Can you work these out from the model? Positions are in its coordinate system, mm. A direction names the side the tool comes from. Give positions to 0.01 mm unless a question says otherwise; leave off trailing zeros. One line per question, with ' | ' between items.
from build123d import *

# Parameters (mm, degrees)
SKETCH1_W             = 25.4
SKETCH1_H             = 25.4
SKETCH1_W_2           = 23.4
SKETCH1_H_2           = 23.4
BOSS_EXTRUDE1_DEPTH   = 304.8
BOSS_EXTRUDE1_2_DEPTH = 304.8
BOSS_EXTRUDE1_3_DEPTH = 304.8
BOSS_EXTRUDE1_4_DEPTH = 304.8
SKETCH2_W             = 25.4
SKETCH2_H             = 25.4
SKETCH2_W_2           = 23.4
SKETCH2_H_2           = 23.4
BOSS_EXTRUDE2_DEPTH   = 508
SKETCH3_W             = 25.4
SKETCH3_H             = 25.4
SKETCH3_W_2           = 23.4
SKETCH3_H_2           = 23.4
BOSS_EXTRUDE4_DEPTH   = 254
LPATTERN2_COUNT       = 2
LPATTERN2_PITCH       = 279.4
SKETCH4_W             = 25.4
SKETCH4_H             = 50.8
SKETCH4_W_2           = 23.4
SKETCH4_H_2           = 48.8
BOSS_EXTRUDE5_DEPTH   = 101.6
SKETCH5_W             = 25.4
SKETCH5_H             = 25.4
SKETCH5_W_2           = 23.4
SKETCH5_H_2           = 23.4
BOSS_EXTRUDE6_DEPTH   = 635
LPATTERN3_COUNT       = 2
LPATTERN3_PITCH       = 660.4
LPATTERN4_COUNT       = 2
LPATTERN4_PITCH       = 736.6


with BuildPart() as part:
    # Sketch1 → Boss-Extrude1 (new body)
    with BuildSketch(Plane(origin=(0, 0, 0), x_dir=(1, 0, 0), z_dir=(0, 1, 0))):
        with Locations((139.7, 266.7)):
            Rectangle(SKETCH1_W, SKETCH1_H)
        with Locations((139.7, 266.7)):
            Rectangle(SKETCH1_W_2, SKETCH1_H_2, mode=Mode.SUBTRACT)
    extrude(amount=BOSS_EXTRUDE1_DEPTH)



with BuildPart() as body_2:
    # Sketch1 → Boss-Extrude1 2 (new body)
    with BuildSketch(Plane(origin=(0, 0, 0), x_dir=(1, 0, 0), z_dir=(0, 1, 0))):
        with Locations((139.7, -266.7)):
            Rectangle(SKETCH1_W, SKETCH1_H)
        with Locations((139.7, -266.7)):
            Rectangle(SKETCH1_W_2, SKETCH1_H_2, mode=Mode.SUBTRACT)
    extrude(amount=BOSS_EXTRUDE1_2_DEPTH)


with BuildPart() as body_3:
    # Sketch1 → Boss-Extrude1 3 (new body)
    with BuildSketch(Plane(origin=(0, 0, 0), x_dir=(1, 0, 0), z_dir=(0, 1, 0))):
        with Locations((-139.7, -266.7)):
            Rectangle(SKETCH1_W, SKETCH1_H)
        with Locations((-139.7, -266.7)):
            Rectangle(SKETCH1_W_2, SKETCH1_H_2, mode=Mode.SUBTRACT)
    extrude(amount=BOSS_EXTRUDE1_3_DEPTH)


with BuildPart() as body_4:
    # Sketch1 → Boss-Extrude1 4 (new body)
    with BuildSketch(Plane(origin=(0, 0, 0), x_dir=(1, 0, 0), z_dir=(0, 1, 0))):
        with Locations((-139.7, 266.7)):
            Rectangle(SKETCH1_W, SKETCH1_H)
        with Locations((-139.7, 266.7)):
            Rectangle(SKETCH1_W_2, SKETCH1_H_2, mode=Mode.SUBTRACT)
    extrude(amount=BOSS_EXTRUDE1_4_DEPTH)


with BuildPart() as part_1:
    add(part.part)

    add(body_2.part)  # Boss-Extrude2 merges body 2
    # Sketch2 → Boss-Extrude2 (add)
    # profile 1 of 2: a face of its own
    with BuildSketch(Plane.XY.offset(-254)):
        with Locations((139.7, 292.1)):
            Rectangle(SKETCH2_W, SKETCH2_H)
        with Locations((139.7, 292.1)):
            Rectangle(SKETCH2_W_2, SKETCH2_H_2, mode=Mode.SUBTRACT)
    # profile 2 of 2: a face of its own
    with BuildSketch(Plane.XY.offset(-254)):
        with Locations((139.7, 12.7)):
            Rectangle(SKETCH2_W, SKETCH2_H)
        with Locations((139.7, 12.7)):
            Rectangle(SKETCH2_W_2, SKETCH2_H_2, mode=Mode.SUBTRACT)
    boss_extrude2 = extrude(amount=BOSS_EXTRUDE2_DEPTH)


    add(body_3.part)  # Boss-Extrude4 merges body 3

    add(body_4.part)  # Boss-Extrude4 merges body 4
    # Sketch3 → Boss-Extrude4 (add)
    # profile 1 of 4: a face of its own
    with BuildSketch(Plane.ZY.offset(-127)):
        with Locations((266.7, 292.1)):
            Rectangle(SKETCH3_W, SKETCH3_H)
        with Locations((266.7, 292.1)):
            Rectangle(SKETCH3_W_2, SKETCH3_H_2, mode=Mode.SUBTRACT)
    # profile 2 of 4: a face of its own
    with BuildSketch(Plane.ZY.offset(-127)):
        with Locations((-266.7, 292.1)):
            Rectangle(SKETCH3_W, SKETCH3_H)
        with Locations((-266.7, 292.1)):
            Rectangle(SKETCH3_W_2, SKETCH3_H_2, mode=Mode.SUBTRACT)
    # profile 3 of 4: a face of its own
    with BuildSketch(Plane.ZY.offset(-127)):
        with Locations((266.7, 12.7)):
            Rectangle(SKETCH3_W, SKETCH3_H)
        with Locations((266.7, 12.7)):
            Rectangle(SKETCH3_W_2, SKETCH3_H_2, mode=Mode.SUBTRACT)
    # profile 4 of 4: a face of its own
    with BuildSketch(Plane.ZY.offset(-127)):
        with Locations((-266.7, 12.7)):
            Rectangle(SKETCH3_W, SKETCH3_H)
        with Locations((-266.7, 12.7)):
            Rectangle(SKETCH3_W_2, SKETCH3_H_2, mode=Mode.SUBTRACT)
    extrude(amount=BOSS_EXTRUDE4_DEPTH)

    # LPattern2: Boss-Extrude2 ×2
    with Locations(*[(-i * LPATTERN2_PITCH, 0, 0) for i in range(1, LPATTERN2_COUNT)]):
        add(boss_extrude2)

    # Sketch4 → Boss-Extrude5 (add)
    # profile 1 of 2: a face of its own
    with BuildSketch(Plane(origin=(0, 0, -279.4), x_dir=(-1, 0, 0), z_dir=(0, 0, -1))):
        with Locations((-139.7, 25.4)):
            Rectangle(SKETCH4_W, SKETCH4_H)
        with Locations((-139.7, 25.4)):
            Rectangle(SKETCH4_W_2, SKETCH4_H_2, mode=Mode.SUBTRACT)
    # profile 2 of 2: a face of its own
    with BuildSketch(Plane(origin=(0, 0, -279.4), x_dir=(-1, 0, 0), z_dir=(0, 0, -1))):
        with Locations((139.7, 25.4)):
            Rectangle(SKETCH4_W, SKETCH4_H)
        with Locations((139.7, 25.4)):
            Rectangle(SKETCH4_W_2, SKETCH4_H_2, mode=Mode.SUBTRACT)
    boss_extrude5 = extrude(amount=BOSS_EXTRUDE5_DEPTH)

    # Sketch5 → Boss-Extrude6 (add)
    # profile 1 of 2: a face of its own
    with BuildSketch(Plane.XZ):
        with Locations((-139.7, -368.3)):
            Rectangle(SKETCH5_W, SKETCH5_H)
        with Locations((-139.7, -368.3)):
            Rectangle(SKETCH5_W_2, SKETCH5_H_2, mode=Mode.SUBTRACT)
    # profile 2 of 2: a face of its own
    with BuildSketch(Plane.XZ):
        with Locations((139.7, -368.3)):
            Rectangle(SKETCH5_W, SKETCH5_H)
        with Locations((139.7, -368.3)):
            Rectangle(SKETCH5_W_2, SKETCH5_H_2, mode=Mode.SUBTRACT)
    boss_extrude6 = extrude(amount=BOSS_EXTRUDE6_DEPTH)

    # LPattern3: Boss-Extrude5 ×2
    with Locations(*[(0, 0, i * LPATTERN3_PITCH) for i in range(1, LPATTERN3_COUNT)]):
        add(boss_extrude5)

    # LPattern4: Boss-Extrude6 ×2
    with Locations(*[(0, 0, i * LPATTERN4_PITCH) for i in range(1, LPATTERN4_COUNT)]):
        add(boss_extrude6)


solid = part_1.part
Q1. On a 3-axis mill with a long thin cutter (end or side, diameter ignored), from which of +Z, -Z, +X, -X, +Y, -Y can I reach the whole of each face in a straight line? I mean faces 1 (the face through (2, 24.4, -267)), 2 (the face through (140, 25, 279.4)), 3 (the face through (-140, 50.8, 331)), 4 (the face through (-140, 1, -329)), 5 (the face through (-140, -313, 355.6)). Say none if no direction works.
Entries:
face 1: none | face 2: +Z | face 3: +Z, +X, -X, +Y | face 4: -Z | face 5: +X, -X, -Y
Q2. If I drill on probe 1 along Z at (x, y) = (134, 49.5); probe 2 along Z at (x, y) = (-139, -236); probe 3 along Y at (x, z) = (-127.5, 217.5), over which ranges is the centre line in solid material (lowest first)? Write a range as from..to.
Entries:
probe 1: -279.4..-278.4, -255..-254, 254..255, 278.4..279.4 | probe 2: -381..-380, -356.6..-355.6, 355.6..356.6, 380..381 | probe 3: 0..25.4, 279.4..304.8
Q3. If we mould it in two halves opening along Y, with no side actions, what happens to faces 6 (the face through (2, 279.4, -267)), 7 (the face through (-140.7, -635, -380.5)), 8 (the face through (140, -313, 380))? For each: pulls with the +Y half, pulls with the -Y half, needs draft (parallel to the pull), parting line crosses it, or undercut.
Entries:
face 6: undercut | face 7: pulls with the -Y half | face 8: needs draft
Q4. For pin 1 Ø11.5 at (x, y) = (135, 196) entering from +Z; pin 2 Ø11.5 at (x, z) = (16.5, -266) entering from -Y; pin 3 Ø18.5 at (x, y) = (134, 16.5) entering from +Z; pin 4 Ø18.5 at (x, y) = (-139, 164) entering from -Z, each with a flat end and sliding along its axis, tell me the tip position at first contact or that it passes through.
Entries:
pin 1: z = 279.4 | pin 2: y = 0 | pin 3: z = 381 | pin 4: z = -279.4
Q5. If we section it at A-A (x = -113): State how many separate pieces and enclosed holes the cut face has, plus the area to 3 significant figures.
Entries:
separate pieces: 4 | enclosed holes: 4 | area: 390 mm²
